Input: part model. Units: mm. Frame: model coordinates. Face numbers are marked on the shaded views. A direction names the side the tool comes from. Round coordinates to 2 decimals unless told otherwise and drop trailing zeros. Order: outer loops, then holes, each group sorted by start corner. A loop starts at its lowest first (then second) coordinate and runs counter-clockwise, first axis right, second up. Notation, with made-up numbers: M 48.25,-31 L 80.25,-31 A15 ccw 80.25,-20 Z; hole C -21,62.5 d1. An arc over 180 degrees is marked long. One line per question, with ' | ' between items.
```python
from build123d import *

# Parameters (mm, degrees)
BOSS_EXTRUDE1_DEPTH = 16
BOSS_EXTRUDE2_DEPTH = 39
SKETCH5_R           = 4
CUT_EXTRUDE1_DEPTH  = 9
SKETCH7_W           = 39
SKETCH7_H           = 16
BOSS_EXTRUDE3_DEPTH = 23
CUT_EXTRUDE2_DEPTH  = 23
SKETCH10_W          = 22
SKETCH10_H          = 4
BOSS_EXTRUDE4_DEPTH = 5


with BuildPart() as part:
    # Sketch2 → Boss-Extrude1 (new body)
    with BuildSketch(Plane(origin=(0, 0, 0), x_dir=(1, 0, 0), z_dir=(0, 1, 0))):
        with BuildLine():
            Line((-15, 43.410987083), (-15, 5.410987083))
            Line((-15, 5.410987083), (15, 5.410987083))
            Line((15, 5.410987083), (15, 43.410987083))
            Line((15, 43.410987083), (7.630797424, 43.410987083))
            Line((7.630797424, 43.410987083), (7.630797424, 20.410987083))
            ThreePointArc((7.630797424, 20.410987083), (0, 12.780189659), (-7.630797424, 20.410987083))
            Line((-7.630797424, 20.410987083), (-7.630797424, 43.410987083))
            Line((-7.630797424, 43.410987083), (-15, 43.410987083))
        make_face()
        with BuildLine():
            ThreePointArc((15, 43.410987083), (0, 58.410987083), (-15, 43.410987083))
            Line((-15, 43.410987083), (-7.630797424, 43.410987083))
            ThreePointArc((-7.630797424, 43.410987083), (0, 51.041784507), (7.630797424, 43.410987083))
            Line((7.630797424, 43.410987083), (15, 43.410987083))
        make_face()
    extrude(amount=-BOSS_EXTRUDE1_DEPTH)



with BuildPart() as body_2:
    # Sketch4 → Boss-Extrude2 (new body)
    with BuildSketch(Plane(origin=(15, 0, 0), x_dir=(0, 0, -1), z_dir=(1, 0, 0))):
        Polygon((5.410987083, 24), (5.410987083, 15), (19.410987083, 15), (19.410987083, 3), (5.410987083, 3), (5.410987083, 0), (28.410987083, 0), (28.410987083, 24), align=None)
    extrude(amount=BOSS_EXTRUDE2_DEPTH)

    # Sketch5 → Cut-Extrude1 (cut)
    with BuildSketch(Plane(origin=(0, 24, 0), x_dir=(1, 0, 0), z_dir=(0, 1, 0))):
        with Locations(Location((27, 13.410987083, 0), (0, 0, 270))):
            Circle(SKETCH5_R)
        with Locations(Location((44, 13.410987083, 0), (0, 0, 270))):
            Circle(SKETCH5_R)
    extrude(amount=-CUT_EXTRUDE1_DEPTH, mode=Mode.SUBTRACT)


with BuildPart() as part_1:
    add(part.part)

    add(body_2.part)  # Boss-Extrude3 merges body 2
    # Sketch7 → Boss-Extrude3 (add)
    with BuildSketch(Plane.XY.offset(-5.410987083)):
        with Locations((34.5, -8)):
            Rectangle(SKETCH7_W, SKETCH7_H)
    extrude(amount=-BOSS_EXTRUDE3_DEPTH)

    # Sketch9 → Cut-Extrude2 (cut)
    with BuildSketch(Plane(origin=(0, 3, 0), x_dir=(1, 0, 0), z_dir=(0, 1, 0))):
        Polygon((21.320508076, 15.410987083), (24, 5.410987083), (45, 5.410987083), (47.679491924, 15.410987083), align=None)
    extrude(amount=-CUT_EXTRUDE2_DEPTH, mode=Mode.SUBTRACT)

    # Sketch10 → Boss-Extrude4 (add)
    with BuildSketch(Plane.XY.offset(-5.410987083)):
        with Locations((0, -18)):
            Rectangle(SKETCH10_W, SKETCH10_H)
    extrude(amount=-BOSS_EXTRUDE4_DEPTH)


solid = part_1.part
```
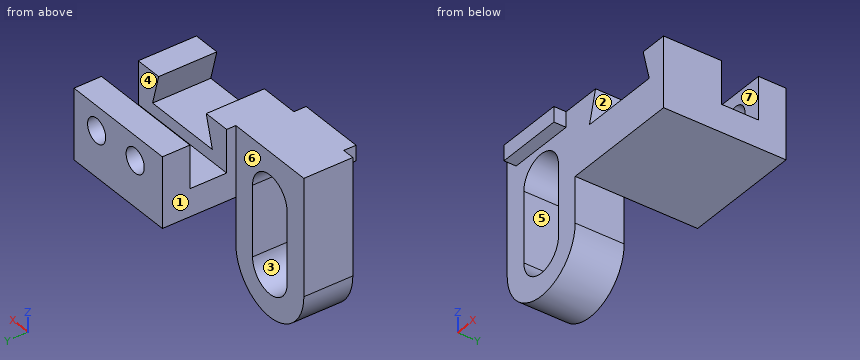
Item 1: First-contact query: pin 1 (11 mm diameter, centred on x = 31.5, z = -11, fed in from -Y); pin 2 (4.5 mm diameter, centred on x = 2.5, y = -17.5, fed in from -Z); pin 3 (7 mm diameter, centred on y = 17.5, z = -18, fed in from -X); pin 4 (1.5 mm diameter, centred on y = 8, z = -17.5, fed in from -X). Flat tips, straight axial feed; report the tip coordinate or a pass-through.
Report:
pin 1: y = -16 | pin 2: z = -58.39 | pin 3: x = 15 | pin 4: through
Item 2: Line query: line 1 along Z through (x, y) = (36.5, 18); line 2 along Z through (x, y) = (42, 13); line 3 along X through (y, z) = (-1, -33). Output: solid intervals per line, ascending. Write a range as from..to.
Report:
line 1: -28.41..-5.41 | line 2: -28.41..-19.41 | line 3: -15..-7.63, 7.63..15
Item 3: Section query C-C, the plane y = -14. Return loops of the section in (x, z).
Report:
outline: M -15,-43.41 A15 ccw 15,-43.41 L 15,-28.41 L 54,-28.41 L 54,-5.41 L 45,-5.41 L 47.68,-15.41 L 21.32,-15.41 L 24,-5.41 L -15,-5.41 Z; hole M -7.63,-43.41 A7.63 ccw 7.63,-43.41 L 7.63,-20.41 A7.63 ccw -7.63,-20.41 Z
Item 4: Section query D-D, the plane x = 36. Return loops of the section in (y, z), plus the area to 3 significant figures.
Report:
outline: M -16,-28.41 L 24,-28.41 L 24,-5.41 L 15,-5.41 L 15,-19.41 L 3,-19.41 L 3,-15.41 L -16,-15.41 Z | area: 562 mm²
Item 5: Section query B-B, the plane z = -22. Return loops of the section in (x, y).
Report:
outline: M -15,-16 L -7.63,-16 L -7.63,0 L -15,0 Z; M 7.63,-16 L 54,-16 L 54,24 L 15,24 L 15,0 L 7.63,0 Z
Item 6: Mould query, pull axis Y, two halves, no side actions, for the marked faces 5, 6 and 7. Classes: +Y half, -Y half, draft (parallel to the pull), parting line (faces both ways), or undercut.
Report:
face 5: draft | face 6: +Y half | face 7: undercut
Item 7: Access query for the marked faces 1, 2, 3 and 4. Directions: +Z, -Z, +X, -X, +Y, -Y. A direction counts if a zero-diameter tool reaches every point of the face in a straight line with its end or side. Return the directions, or none.
Report:
face 1: +Z, -Z, -X, +Y | face 2: -Y | face 3: +Y, -Y | face 4: +Z, +X, -X
Item 8: Section query A-A, the plane x = 27. Return loops of the section in (y, z).
Report:
outline: M -16,-28.41 L 24,-28.41 L 24,-17.41 L 15,-17.41 L 15,-19.41 L 3,-19.41 L 3,-15.41 L -16,-15.41 Z; M 15,-9.41 L 24,-9.41 L 24,-5.41 L 15,-5.41 Z
